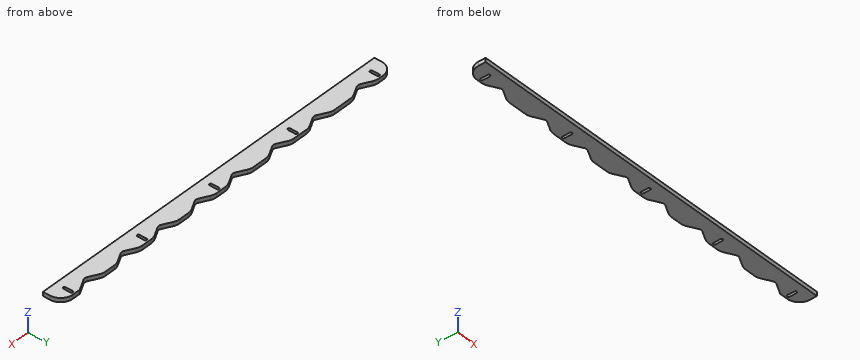
from build123d import *

# Parameters (mm, degrees)
RESSALTO_EXTRUS_O1_DEPTH = 20


with BuildPart() as part:
    # Esboço1 → Ressalto-extrusão1 (new body)
    # profile 1 of 2: a face of its own
    with BuildSketch(Plane.XY):
        with BuildLine():
            Line((-938.823833844, -27.471849847), (-938.823833844, -32.471849847))
            Line((-938.823833844, -32.471849847), (-936.823833844, -32.471849847))
            Line((-936.823833844, -32.471849847), (941.176166156, -32.471849847))
            Line((941.176166156, -32.471849847), (941.176166156, -27.471849847))
            ThreePointArc((941.176166156, -27.471849847), (923.602573027, 14.954557024), (881.176166156, 32.528150153))
            Line((881.176166156, 32.528150153), (846.261701379, 32.528150153))
            Line((846.261701379, 32.528150153), (842.001592443, 32.528150153))
            Line((842.001592443, 32.528150153), (785.565597412, 2.52059931))
            ThreePointArc((785.565597412, 2.52059931), (776.176166156, 0.179551167), (766.7867349, 2.52059931))
            Line((766.7867349, 2.52059931), (723.559353465, 25.505005725))
            ThreePointArc((723.559353465, 25.505005725), (709.906373434, 30.74589373), (695.391059698, 32.528150153))
            Line((695.391059698, 32.528150153), (646.961272614, 32.528150153))
            ThreePointArc((646.961272614, 32.528150153), (632.445958878, 30.74589373), (618.792978847, 25.505005725))
            Line((618.792978847, 25.505005725), (575.565597412, 2.52059931))
            ThreePointArc((575.565597412, 2.52059931), (566.176166156, 0.179551167), (556.7867349, 2.52059931))
            Line((556.7867349, 2.52059931), (513.559353465, 25.505005725))
            ThreePointArc((513.559353465, 25.505005725), (499.906373434, 30.74589373), (485.391059698, 32.528150153))
            Line((485.391059698, 32.528150153), (436.961272614, 32.528150153))
            ThreePointArc((436.961272614, 32.528150153), (422.445958878, 30.74589373), (408.792978847, 25.505005725))
            Line((408.792978847, 25.505005725), (365.565597412, 2.52059931))
            ThreePointArc((365.565597412, 2.52059931), (356.176166156, 0.179551167), (346.7867349, 2.52059931))
            Line((346.7867349, 2.52059931), (303.559353465, 25.505005725))
            ThreePointArc((303.559353465, 25.505005725), (289.906373434, 30.74589373), (275.391059698, 32.528150153))
            Line((275.391059698, 32.528150153), (226.961272614, 32.528150153))
            ThreePointArc((226.961272614, 32.528150153), (212.445958878, 30.74589373), (198.792978847, 25.505005725))
            Line((198.792978847, 25.505005725), (155.565597412, 2.52059931))
            ThreePointArc((155.565597412, 2.52059931), (146.176166156, 0.179551167), (136.7867349, 2.52059931))
            Line((136.7867349, 2.52059931), (93.559353465, 25.505005725))
            ThreePointArc((93.559353465, 25.505005725), (79.906373434, 30.74589373), (65.391059698, 32.528150153))
            Line((65.391059698, 32.528150153), (16.961272614, 32.528150153))
            ThreePointArc((16.961272614, 32.528150153), (2.445958878, 30.74589373), (-11.207021153, 25.505005725))
            Line((-11.207021153, 25.505005725), (-54.434402588, 2.52059931))
            ThreePointArc((-54.434402588, 2.52059931), (-63.823833844, 0.179551167), (-73.2132651, 2.52059931))
            Line((-73.2132651, 2.52059931), (-116.440646535, 25.505005725))
            ThreePointArc((-116.440646535, 25.505005725), (-130.093626566, 30.74589373), (-144.608940302, 32.528150153))
            Line((-144.608940302, 32.528150153), (-213.038727386, 32.528150153))
            ThreePointArc((-213.038727386, 32.528150153), (-227.554041122, 30.74589373), (-241.207021153, 25.505005725))
            Line((-241.207021153, 25.505005725), (-284.434402588, 2.52059931))
            ThreePointArc((-284.434402588, 2.52059931), (-293.823833844, 0.179551167), (-303.2132651, 2.52059931))
            Line((-303.2132651, 2.52059931), (-346.440646535, 25.505005725))
            ThreePointArc((-346.440646535, 25.505005725), (-360.093626566, 30.74589373), (-374.608940302, 32.528150153))
            Line((-374.608940302, 32.528150153), (-443.038727386, 32.528150153))
            ThreePointArc((-443.038727386, 32.528150153), (-457.554041122, 30.74589373), (-471.207021153, 25.505005725))
            Line((-471.207021153, 25.505005725), (-514.434402588, 2.52059931))
            ThreePointArc((-514.434402588, 2.52059931), (-523.823833844, 0.179551167), (-533.2132651, 2.52059931))
            Line((-533.2132651, 2.52059931), (-576.440646535, 25.505005725))
            ThreePointArc((-576.440646535, 25.505005725), (-590.093626566, 30.74589373), (-604.608940302, 32.528150153))
            Line((-604.608940302, 32.528150153), (-693.038727386, 32.528150153))
            ThreePointArc((-693.038727386, 32.528150153), (-707.554041122, 30.74589373), (-721.207021153, 25.505005725))
            Line((-721.207021153, 25.505005725), (-764.434402588, 2.52059931))
            ThreePointArc((-764.434402588, 2.52059931), (-773.823833844, 0.179551167), (-783.2132651, 2.52059931))
            Line((-783.2132651, 2.52059931), (-826.440646535, 25.505005725))
            ThreePointArc((-826.440646535, 25.505005725), (-840.093626566, 30.74589373), (-854.608940302, 32.528150153))
            Line((-854.608940302, 32.528150153), (-878.823833844, 32.528150153))
            ThreePointArc((-878.823833844, 32.528150153), (-921.250240715, 14.954557024), (-938.823833844, -27.471849847))
        make_face()
        with BuildLine():
            ThreePointArc((-875.073833844, 17.528150153), (-868.823833844, 23.778150153), (-862.573833844, 17.528150153))
            Line((-862.573833844, 17.528150153), (-862.573833844, -17.471849847))
            ThreePointArc((-862.573833844, -17.471849847), (-868.823833844, -23.721849847), (-875.073833844, -17.471849847))
            Line((-875.073833844, -17.471849847), (-875.073833844, 17.528150153))
        make_face(mode=Mode.SUBTRACT)
        with BuildLine():
            ThreePointArc((-410.073833844, 17.528150153), (-403.823833844, 23.778150153), (-397.573833844, 17.528150153))
            Line((-397.573833844, 17.528150153), (-397.573833844, -17.471849847))
            ThreePointArc((-397.573833844, -17.471849847), (-403.823833844, -23.721849847), (-410.073833844, -17.471849847))
            Line((-410.073833844, -17.471849847), (-410.073833844, 17.528150153))
        make_face(mode=Mode.SUBTRACT)
        with BuildLine():
            ThreePointArc((47.426166156, -17.471849847), (41.176166156, -23.721849847), (34.926166156, -17.471849847))
            Line((34.926166156, -17.471849847), (34.926166156, 17.528150153))
            ThreePointArc((34.926166156, 17.528150153), (41.176166156, 23.778150153), (47.426166156, 17.528150153))
            Line((47.426166156, 17.528150153), (47.426166156, -17.471849847))
        make_face(mode=Mode.SUBTRACT)
        with BuildLine():
            ThreePointArc((444.926166156, 17.528150153), (451.176166156, 23.778150153), (457.426166156, 17.528150153))
            Line((457.426166156, 17.528150153), (457.426166156, -17.471849847))
            ThreePointArc((457.426166156, -17.471849847), (451.176166156, -23.721849847), (444.926166156, -17.471849847))
            Line((444.926166156, -17.471849847), (444.926166156, 17.528150153))
        make_face(mode=Mode.SUBTRACT)
        with BuildLine():
            ThreePointArc((877.426166156, -17.471849847), (871.176166156, -23.721849847), (864.926166156, -17.471849847))
            Line((864.926166156, -17.471849847), (864.926166156, 17.528150153))
            ThreePointArc((864.926166156, 17.528150153), (871.176166156, 23.778150153), (877.426166156, 17.528150153))
            Line((877.426166156, 17.528150153), (877.426166156, -17.471849847))
        make_face(mode=Mode.SUBTRACT)
    # profile 2 of 2: a face of its own
    with BuildSketch(Plane.XY):
        Polygon((-936.823833844, -32.471849847), (-938.823833844, -32.471849847), (-938.823833844, -62.471849847), (941.176166156, -62.471849847), (941.176166156, -32.471849847), align=None)
    extrude(amount=RESSALTO_EXTRUS_O1_DEPTH)


solid = part.part
Read the model definition and answer for the solid it produces. Units are mm, in the model's axes. Round coordinates to 2 decimals unless told otherwise and drop trailing zeros. Order: outer loops, then holes, each group sorted by start corner. A loop starts at its lowest first (then second) coordinate and runs counter-clockwise, first axis right, second up. Notation, with made-up numbers: (84.5, -16.5) - (112.5, -16.5) arc R23 cw to (112.5, 12.5) - close; hole circle Ø5 at (87.5, -28). An arc over 180 degrees is marked (long way). Use one line per item in the form item = value. Start each with the question number.
(1) Find the intervals of material crossed by line 1 along X through (y, z) = (-9, 1.75); line 2 along X through (y, z) = (-7.5, 13.5); line 3 along X through (y, z) = (-26, 17.25), in increasing order. Write a range as from..to.
(2) The part is cut by section B-B (x = 389). Give the vertices of the cut face in (y, z), then the cut area to 3 significant figures.
(3) The part is cut by section A-A (z = 6). Count the separate pieces of the cut face and the enclosed holes in it, then the cut area to 3 significant figures.
(4) The part is cut by section C-C (x = 596). Give the vertices of the cut face in (y, z).
(5) Flat-ended cylindrical pins translate along their axes: pin 1 Ø10 at (x, z) = (-466.5, 8) entering from +Y; pin 2 Ø10 at (y, z) = (-0.5, 7.5) entering from -X; pin 3 Ø6 at (y, z) = (8.5, 6) entering from -X. Find the tip coordinate at first contact, or state that the pin passes through.
Checked values:
q1.line_1 = -935.91..-875.07, -862.57..-410.07, -397.57..34.93, 47.43..444.93, 457.43..864.93, 877.43..938.26
q1.line_2 = -935.4..-875.07, -862.57..-410.07, -397.57..34.93, 47.43..444.93, 457.43..864.93, 877.43..937.75
q1.line_3 = -938.81..941.16
q2.outline = (-62.47, 0) - (14.98, 0) - (14.98, 20) - (-62.47, 20) - close
q2.area = 1,550 mm^2
q3.separate_pieces = 1
q3.enclosed_holes = 5
q3.area = 156,000 mm^2
q4.outline = (-62.47, 0) - (13.39, 0) - (13.39, 20) - (-62.47, 20) - close
q5.pin_1 = 29.62
q5.pin_2 = -934.66
q5.pin_3 = -928.95
